Here's how the part is built. I have some questions about the finished solid (model axes, mm). Coordinates: 2 decimals unless noted, no trailing zeros. Write each loop counter-clockwise with the first axis right and the second up, starting at its lowest first coordinate (ties: lowest second). Pieces come first, ordered by that corner, then holes.
Item 1: If we section it at A-A (y = 0): Please give me the cut outline in (x, z), then the cut area to 3 significant figures.
Item 2: If I drill on line 1 (Z direction, x = 9, y = 0.5); line 2 (Z direction, x = 2.5, y = 3.5); line 3 (Y direction, x = 13.75, z = 0), over which ranges is the centre line in solid material (lowest first)?
Item 3: If we section it at B-B (z = 0): Please give me the cut outline in (x, y), then the cut area to 3 significant figures.
Item 4: If we section it at C-C (z = 15.5): Please give me the cut outline in (x, y).
Item 5: I'm going to push flat-ended pins straight in: pin 1 Ø4 at (x, z) = (6.5, -10) entering from +Y; pin 2 Ø17 at (y, z) = (0, 0) entering from +X; pin 3 Ø8 at (y, z) = (4.5, 11.5) entering from +X; pin 4 Ø4 at (x, z) = (2.5, 9.5) entering from +Y. Where does each tip first touch, or does it pass through?
Item 6: We'd pull the mould along Z, two halves only. Please class faces 1 (the face through (10.02, -15.89, -20.77)), 2 (the face through (10.018, 10.066, 24.084)), 3 (the face through (10.02, -23.31, 13.6)): +Z half, -Z half, draft (parallel to the pull), parting line (faces both ways), or undercut.
from build123d import *

# Parameters (mm, degrees)
SKETCH1_R           = 14.2875
BOSS_EXTRUDE1_DEPTH = 20.32


with BuildPart() as part:
    # Sketch1 → Boss-Extrude1 (new body)
    with BuildSketch(Plane(origin=(0, 0, 0), x_dir=(0, 0, -1), z_dir=(1, 0, 0))):
        with BuildLine():
            Line((-2.413, 23.8125), (-2.413, 23.940510589))
            ThreePointArc((-2.413, 23.940510589), (-3.349172921, 25.91011428), (-5.467597403, 26.427836364))
            ThreePointArc((-5.467597403, 26.427836364), (-13.49375, 23.371860585), (-20.153378957, 17.94899643))
            ThreePointArc((-20.153378957, 17.94899643), (-20.764230721, 15.855525972), (-19.526590349, 14.059974594))
            Line((-19.526590349, 14.059974594), (-19.415729928, 13.995969299))
            ThreePointArc((-19.415729928, 13.995969299), (-18.532510628, 10.69975), (-21.828729928, 9.816530701))
            Line((-21.828729928, 9.816530701), (-21.939590349, 9.880535995))
            ThreePointArc((-21.939590349, 9.880535995), (-24.113403642, 10.054588309), (-25.62097636, 8.478839934))
            ThreePointArc((-25.62097636, 8.478839934), (-26.9875, 0), (-25.62097636, -8.478839934))
            ThreePointArc((-25.62097636, -8.478839934), (-24.113403642, -10.054588309), (-21.939590349, -9.880535995))
            Line((-21.939590349, -9.880535995), (-21.828729928, -9.816530701))
            ThreePointArc((-21.828729928, -9.816530701), (-18.532510628, -10.69975), (-19.415729928, -13.995969299))
            Line((-19.415729928, -13.995969299), (-19.526590349, -14.059974594))
            ThreePointArc((-19.526590349, -14.059974594), (-20.764230721, -15.855525972), (-20.153378957, -17.94899643))
            ThreePointArc((-20.153378957, -17.94899643), (-13.49375, -23.371860585), (-5.467597403, -26.427836364))
            ThreePointArc((-5.467597403, -26.427836364), (-3.349172921, -25.91011428), (-2.413, -23.940510589))
            Line((-2.413, -23.940510589), (-2.413, -23.8125))
            ThreePointArc((-2.413, -23.8125), (0, -21.3995), (2.413, -23.8125))
            Line((2.413, -23.8125), (2.413, -23.940510589))
            ThreePointArc((2.413, -23.940510589), (3.349172921, -25.91011428), (5.467597403, -26.427836364))
            ThreePointArc((5.467597403, -26.427836364), (13.49375, -23.371860585), (20.153378957, -17.94899643))
            ThreePointArc((20.153378957, -17.94899643), (20.764230721, -15.855525972), (19.526590349, -14.059974594))
            Line((19.526590349, -14.059974594), (19.415729928, -13.995969299))
            ThreePointArc((19.415729928, -13.995969299), (18.532510628, -10.69975), (21.828729928, -9.816530701))
            Line((21.828729928, -9.816530701), (21.939590349, -9.880535995))
            ThreePointArc((21.939590349, -9.880535995), (24.113403642, -10.054588309), (25.62097636, -8.478839934))
            ThreePointArc((25.62097636, -8.478839934), (26.9875, 0), (25.62097636, 8.478839934))
            ThreePointArc((25.62097636, 8.478839934), (24.113403642, 10.054588309), (21.939590349, 9.880535995))
            Line((21.939590349, 9.880535995), (21.828729928, 9.816530701))
            ThreePointArc((21.828729928, 9.816530701), (18.532510628, 10.69975), (19.415729928, 13.995969299))
            Line((19.415729928, 13.995969299), (19.526590349, 14.059974594))
            ThreePointArc((19.526590349, 14.059974594), (20.764230721, 15.855525972), (20.153378957, 17.94899643))
            ThreePointArc((20.153378957, 17.94899643), (13.49375, 23.371860585), (5.467597403, 26.427836364))
            ThreePointArc((5.467597403, 26.427836364), (3.349172921, 25.91011428), (2.413, 23.940510589))
            Line((2.413, 23.940510589), (2.413, 23.8125))
            ThreePointArc((2.413, 23.8125), (0, 21.3995), (-2.413, 23.8125))
        make_face()
        Circle(SKETCH1_R, mode=Mode.SUBTRACT)
    extrude(amount=BOSS_EXTRUDE1_DEPTH)


solid = part.part
Answer list:
1. outline: (0, -26.99) - (20.32, -26.99) - (20.32, -14.29) - (0, -14.29) - close; (0, 14.29) - (20.32, 14.29) - (20.32, 26.99) - (0, 26.99) - close
1. area: 516 mm2
2. line 1: z = -26.98 to -14.28, 14.28 to 26.98
2. line 2: z = -26.76 to -13.85, 13.85 to 26.76
2. line 3: y = -21.4 to -14.29, 14.29 to 21.4
3. outline: (0, -21.4) - (20.32, -21.4) - (20.32, -14.29) - (0, -14.29) - close; (0, 14.29) - (20.32, 14.29) - (20.32, 21.4) - (0, 21.4) - close
3. area: 289 mm2
4. outline: (0, -22.09) - (20.32, -22.09) - (20.32, 22.09) - (0, 22.09) - close
5. pin 1: stops at y = 25.77
5. pin 2: passes through
5. pin 3: stops at x = 20.32
5. pin 4: stops at y = 25.92
6. face 1: -Z half
6. face 2: undercut
6. face 3: +Z half
